from build123d import *

# Parameters (mm, degrees)
F0_W     = 36
F0_H     = 68
F1_DEPTH = 652
F3_DEPTH = 36
F4_W     = 68
F4_H     = 68
F5_DEPTH = 18
F7_DEPTH = 18


with BuildPart() as f1:
    # F0 (on Front) → F1 (new body)
    with BuildSketch(Plane.XZ):
        Rectangle(F0_W, F0_H)
    extrude(amount=F1_DEPTH)

    # F2 (on face) → F3 (cut, through all)
    with BuildSketch(Plane.YZ.offset(18)):
        Polygon((0, -34), (0, 34), (-18.220545, -34), align=None)
    extrude(amount=-F3_DEPTH, mode=Mode.SUBTRACT)

    # F4 (on face) → F5 (cut)
    with BuildSketch(Plane.YZ.offset(18)):
        with Locations((-618, 0)):
            Rectangle(F4_W, F4_H)
    extrude(amount=-F5_DEPTH, mode=Mode.SUBTRACT)

    # F6 (on face) → F7 (cut)
    with BuildSketch(Plane.YZ.offset(18)):
        Polygon((-183.5, 34), (-254, 34), (-235.779455, -34), (-165.279455, -34), align=None)
    extrude(amount=-F7_DEPTH, mode=Mode.SUBTRACT)


solid = f1.part
The model under review builds one solid part; all positions refer to its coordinate system, in mm. A direction names the side the tool comes from. Give positions to 0.01 mm unless a question says otherwise; leave off trailing zeros. Loops run counter-clockwise (first coordinate to the right, second up) from the corner with the lowest first, then second, coordinate; pieces in that order, holes last. Notation, with made-up numbers: (-28.5, 54) -> (-11.5, 54) arc R13 ccw to (-11.5, 61) -> close; hole circle Ø5 at (-38.75, 4.25). An arc over 180 degrees is marked (long way). Answer as a JSON object with one key per item and string values. Group by question number.
Q1. Tool access review of faces 1 (the flat face through (9, -584, 0)), 2 (the flat face through (9.13, -245.02, 0.48)), 3 (the flat face through (0, -210, 0)): name each direction out of +Z, -Z, +X, -X, +Y, -Y from which nothing blocks a thin tool from reaching the whole face with its end or side.
Q2. Take a section at A-A (x = 8). Write out the cut boundary in (y, z).
Q3. Wall thickness on line 1 along X through (y, z) = (-173, -10.5); line 2 along Y through (x, z) = (5.5, -19.5); line 3 along Y through (x, z) = (6.5, 14): over which ranges is each line inside the solid? List them lowest first.
Q4. Take a section at B-B (z = 10.5). Write out the cut boundary in (x, y).
Q5. Take a section at C-C (y = -216). Write out the cut boundary in (x, z).
Q6. Insertion check: pin 1 (5 mm diameter, centred on x = 12, z = -1, fed in from -Y); pin 2 (20.5 mm diameter, centred on y = -606, z = 7, fed in from +X); pin 3 (8 mm diameter, centred on x = -6.5, z = 3, fed in from +Y). Each pin has a flat end and moves straight along its axis. Give the tip position at first contact, or say it passes through.
Q7. Draft analysis for pull direction Y (two halves, no side actions). For faces 4 (the flat face through (-9, -652, 0)), 5 (the flat face through (18, -90, 0)), 6 (the flat face through (0.25, -8.98, 0.48)), 7 (the flat face through (9.13, -174.26, -0.48)), state which applies: pulls with the +Y half, pulls with the -Y half, needs draft (parallel to the pull), parting line crosses it, or undercut.
Q8. Take a section at D-D (z = -17). Write out the cut boundary in (x, y).
Answer below:
{
 "1": {"face 1": "+Z, -Z, +X, -Y", "face 2": "+Z, +X", "face 3": "+X"},
 "2": {"outline": "(-584, -34) -> (-235.78, -34) -> (-254, 34) -> (-584, 34) -> close; (-183.5, 34) -> (-165.28, -34) -> (-18.22, -34) -> (0, 34) -> close"},
 "3": {"line 1": "x = -18 to 0", "line 2": "y = -584 to -239.66, -169.16 to -14.34", "line 3": "y = -584 to -248.64, -178.14 to -5.36"},
 "4": {"outline": "(-18, -652) -> (0, -652) -> (0, -584) -> (18, -584) -> (18, -247.7) -> (0, -247.7) -> (0, -177.2) -> (18, -177.2) -> (18, -6.3) -> (-18, -6.3) -> close"},
 "5": {"outline": "(-18, -34) -> (0, -34) -> (0, 34) -> (-18, 34) -> close"},
 "6": {"pin 1": "stops at y = -584", "pin 2": "stops at x = 0", "pin 3": "stops at y = -7.23"},
 "7": {"face 4": "pulls with the -Y half", "face 5": "needs draft", "face 6": "pulls with the +Y half", "face 7": "undercut"},
 "8": {"outline": "(-18, -652) -> (0, -652) -> (0, -584) -> (18, -584) -> (18, -240.33) -> (0, -240.33) -> (0, -169.83) -> (18, -169.83) -> (18, -13.67) -> (-18, -13.67) -> close"}
}
